The model under review builds one solid part; all positions refer to its coordinate system, in mm. A direction names the side the tool comes from. Coordinates: 2 decimals unless noted, no trailing zeros. Write each loop counter-clockwise with the first axis right and the second up, starting at its lowest first coordinate (ties: lowest second). Pieces come first, ordered by that corner, then holes.
1) Add section C-C, the plane z = 48. State the section outline as (x, y) points.
2) Add section A-A, the plane z = -240.5. Give the number of separate pieces and of enclosed holes in the cut face, then the cut area to 3 significant figures.
3) For P1, Ø9, axis at x = 32, y = 309.5, coming from the -Z side; P2, Ø4, axis at y = 41.5, z = -167.5, coming from the -X side; P3, Ø8, axis at y = 70.5, z = -245, coming from the +X side, all flat-tipped, find the tip position at first contact; note any pin that passes through.
4) For line 1 (Y direction, x = 110, z = -224); line 2 (Z direction, x = 26, y = 167.5); line 3 (Z direction, x = 50, y = -38.5), list the stretches that pass through material, from the lowest coordinate up.
5) Machinability: for faces 1 (the cylindrical face through (113.3, -105.3, -225)), 2 (the cylindrical face through (69.02, 15.521, -67.573)), 3 (the flat face through (140, 96, -146)), 4 (the flat face through (130, 115, -193)), which of the approach directions +Z, -Z, +X, -X, +Y, -Y give a long, thin tool a straight path to every point of the face, cutting with its end or side? Answer none if there is none.
6) Add section B-B, the plane x = 110. State the section outline as (y, z) points.
7) Mouldability with a two-part tool opening along Z and no side actions: class faces 5 (the flat face through (69, 344.798, -149)), 6 (the cylindrical face through (69.02, 16.104, 67.764)), 7 (the flat face through (110, -90, -153.998)) as released by +Z, released by -Z, zero draft, split by the parting line, or undercut.
from build123d import *

# Parameters (mm, degrees)
BOSS_EXTRUDE1_DEPTH = 140
SKETCH2_R           = 15
CUT_EXTRUDE1_DEPTH  = 140
CUT_EXTRUDE2_START  = -10
CUT_EXTRUDE2_DEPTH  = 10
CUT_EXTRUDE3_DEPTH  = 10
FILLET1_R           = 10


with BuildPart() as part:
    # Sketch1 → Boss-Extrude1 (new body)
    with BuildSketch(Plane(origin=(0, 0, 0), x_dir=(0, 0, -1), z_dir=(1, 0, 0))):
        with BuildLine():
            Line((0, -120.66577438), (293.9982389, -120.66577438))
            Line((293.9982389, -120.66577438), (293.9982389, 344.79792692))
            Line((293.9982389, 344.79792692), (0, 344.79792692))
            ThreePointArc((0, 344.79792692), (-166.188863738, 217.33208751), (-86.160329475, 23.781803731))
            ThreePointArc((-86.160329475, 23.781803731), (-77.169593528, 12.698658653), (-77.855834661, -1.556112857))
            ThreePointArc((-77.855834661, -1.556112857), (-71.148862357, -82.172111425), (0, -120.66577438))
        make_face()
        with BuildLine():
            ThreePointArc((81.153066922, 32.43786067), (0, 334.79792692), (-81.153066922, 32.43786067))
            ThreePointArc((-81.153066922, 32.43786067), (-67.666963002, 15.813143052), (-68.696324701, -5.569014213))
            ThreePointArc((-68.696324701, -5.569014213), (0, -110.66577438), (68.696324701, -5.569014213))
            ThreePointArc((68.696324701, -5.569014213), (67.666963002, 15.813143052), (81.153066922, 32.43786067))
        make_face(mode=Mode.SUBTRACT)
    extrude(amount=BOSS_EXTRUDE1_DEPTH)

    # Sketch2 → Cut-Extrude1 (cut)
    with BuildSketch(Plane(origin=(0, 0, -293.9982389), x_dir=(-1, 0, 0), z_dir=(0, 0, -1))):
        with Locations((-110, 314.79792692)):
            Circle(SKETCH2_R)
        with Locations((-30, -90.66577438)):
            Circle(SKETCH2_R)
        with Locations((-110, -90.66577438)):
            Circle(SKETCH2_R)
        with Locations((-30, 314.79792692)):
            Circle(SKETCH2_R)
    extrude(amount=-CUT_EXTRUDE1_DEPTH, mode=Mode.SUBTRACT)

    # Sketch3 → Cut-Extrude2 (cut)
    with BuildSketch(Plane(origin=(140, 0, 0), x_dir=(0, 0, -1), z_dir=(1, 0, 0)).offset(CUT_EXTRUDE2_START)):
        with BuildLine():
            Line((40, -110.66577438), (283.9982389, -110.66577438))
            Line((283.9982389, -110.66577438), (283.9982389, 334.79792692))
            Line((283.9982389, 334.79792692), (57.804969406, 334.79792692))
            ThreePointArc((57.804969406, 334.79792692), (171.360027548, 188.350107316), (86.160329475, 23.781803731))
            ThreePointArc((86.160329475, 23.781803731), (77.169593528, 12.698658653), (77.855834661, -1.556112857))
            ThreePointArc((77.855834661, -1.556112857), (80.303978733, -63.527414671), (40, -110.66577438))
        make_face()
    extrude(amount=CUT_EXTRUDE2_DEPTH, mode=Mode.SUBTRACT)

    # Sketch4 → Cut-Extrude3 (cut)
    with BuildSketch(Plane.ZY):
        with BuildLine():
            Line((-57.804969406, 334.79792692), (-283.9982389, 334.79792692))
            Line((-283.9982389, 334.79792692), (-283.9982389, -110.66577438))
            Line((-283.9982389, -110.66577438), (-40, -110.66577438))
            ThreePointArc((-40, -110.66577438), (-80.303978733, -63.527414671), (-77.855834661, -1.556112857))
            ThreePointArc((-77.855834661, -1.556112857), (-77.169593528, 12.698658653), (-86.160329475, 23.781803731))
            ThreePointArc((-86.160329475, 23.781803731), (-171.360027548, 188.350107316), (-57.804969406, 334.79792692))
        make_face()
    extrude(amount=-CUT_EXTRUDE3_DEPTH, mode=Mode.SUBTRACT)

    # Fillet1
    fillet1_edges = [part.edges().sort_by_distance(p)[0] for p in [
        (130, 334.79792692, -170.901604153),
        (130, 112.06607627, -283.9982389),
        (130, -110.66577438, -161.99911945),
        (130, -63.527414671, -80.303978733),
        (130, 12.698658653, -77.169593528),
        (130, 188.350107316, -171.360027548),
        (10, 12.698658653, -77.169593528),
        (10, -63.527414671, -80.303978733),
        (10, -110.66577438, -161.99911945),
        (10, 112.06607627, -283.9982389),
        (10, 334.79792692, -170.901604153),
        (10, 188.350107316, -171.360027548),
    ]]
    fillet(fillet1_edges, radius=FILLET1_R - 0.0001)  # a hair under: the kernel refuses the full size


solid = part.part
Geometry results:
1. outline: (0, -105.82) - (140, -105.82) - (140, -93.29) - (0, -93.29) - close; (0, 327.53) - (140, 327.53) - (140, 337.97) - (0, 337.97) - close
2. separate pieces: 1
2. enclosed holes: 4
2. area: 53,500 mm2
3. P1: stops at z = -154
3. P2: stops at x = 10
3. P3: stops at x = 130
4. line 1: y = -120.67 to -105.67, -75.67 to 299.8, 329.8 to 344.8
4. line 2: z = -294 to -161.99, 161.99 to 171.99
4. line 3: z = -294 to -74.95, 74.95 to 84.95
5. face 1: -Z
5. face 2: +X, -X
5. face 3: +Z, -Z, +X, +Y, -Y
5. face 4: +X
6. outline: (-120.67, -294) - (-105.67, -294) - (-105.67, -154) - (-75.67, -154) - (-75.67, -294) - (299.8, -294) - (299.8, -154) - (329.8, -154) - (329.8, -294) - (344.8, -294) - (344.8, 0) arc R172.07 ccw to (23.78, 86.16) arc R20 cw to (-1.56, 77.86) arc R85 ccw to (-120.67, 0) - close; hole (-5.57, -68.7) arc R30 cw to (32.44, -81.15) arc R162.07 ccw (long way) to (32.44, 81.15) arc R30 cw to (-5.57, 68.7) arc R75 ccw (long way) to start
7. face 5: zero draft
7. face 6: undercut
7. face 7: released by -Z
